Source: CAD feature listing. Evaluate the final solid. Frame: model axes, mm. A direction names the side the tool comes from. Coordinates: 2 decimals unless noted, no trailing zeros. Write each loop counter-clockwise with the first axis right and the second up, starting at its lowest first coordinate (ties: lowest second). Pieces come first, ordered by that corner, then holes. Notation, with made-up numbers: M 52.25,81 L 62.25,81 A16 ccw 62.25,107 Z; hole C 86.25,38 d5. An arc over 180 degrees is marked long. One line per item, written item: value. Start each with the question number.
Item 1: Cut plane B-B, the plane y = 30.25. Output: boundary loops of the cut face in (x, z) (3 decimals), then the cut area to 3 significant figures.
Item 2: Cut plane A-A, the plane x = 0. State how many separate pieces and enclosed holes the cut face has, then the cut area to 3 significant figures.
Item 3: Mould query, pull axis Z, two halves, no side actions, for faces 1 (the cylindrical face through (1, 26, 0)), 2 (the cylindrical face through (2.4, 30.7, -0.5)), 3 (the flat face through (3, 23.4, 0)). Classes: released by +Z, released by -Z, zero draft, split by the parting line, or undercut.
Item 4: Ray query, L1, parallel to Z at x = 0, y = 20.2; L2, parallel to Z at x = 0, y = 29.5; L3, parallel to Z at x = 0, y = 26 (3 decimals). Return the intervals inside material, ascending. Write a range as from..to.
Item 5: Cut plane C-C, the plane y = 22.5. Output: boundary loops of the cut face in (x, z), then the cut area to 3 significant figures.
Item 6: Pin query (flat end, axial travel): P1, Ø2, axis at x = -5, z = 0, coming from the +Y side; P2, Ø1.1, axis at x = 0, z = 5, coming from the +Y side; P3, Ø4, axis at y = 21, z = -4, coming from the +X side; P4, Ø2, axis at y = 22.5, z = -3, coming from the -X side. Return the tip coordinate at first contact, or that it passes through.
Item 7: Set-up query: faces 4 (the cylindrical face through (2.4, 28.2, -0.5)), 5 (the cylindrical face through (-1.792, 30.094, 1.142)), 6 (the cylindrical face through (-2.85, 19.59, -0.37)). Return all of +Z, -Z, +X, -X, +Y, -Y with unobstructed straight access to the full face (end or side cutting, diameter ignored); none if empty.
Item 8: Cut plane D-D, the plane y = 24. Output: boundary loops of the cut face in (x, z), then the cut area to 3 significant figures.
Autodesk Inventor part; units mm, degrees
ref_plane "Work Plane8" through (0, 26.3, 0) normal (0, 1, 0) x (1, 0, 0)
ref_plane "Work Plane9" through (0, 30.1, 0) normal (0, 1, 0) x (1, 0, 0)
ref_plane "YZ Plane" through (0, 0, 0) normal (1, 0, 0) x (0, 1, 0)
sketch "Sketch1" plane through (0, 0, 0) normal (1, 0, 0) x (0, 1, 0)
  line L0 (31, 0) -> (20.4, 0)
  line L1 (31, 0) -> (32, 0)
  line L2 (32, 0) -> (32, 2.45)
  line L3 (32, 2.45) -> (30.5, 2.45)
  line L4 (30.5, 2.45) -> (30.5, 2.125)
  line L5 (30.5, 2.125) -> (29.7, 2.125)
  line L6 (29.7, 2.125) -> (29.7, 2.45)
  line L7 (29.7, 2.45) -> (26.7, 2.45)
  line L8 (26.7, 2.45) -> (26.7, 2.125)
  line L9 (26.7, 2.125) -> (25.9, 2.125)
  line L10 (25.9, 2.125) -> (25.9, 2.45)
  line L11 (25.9, 2.45) -> (24.4, 2.45)
  line L12 (23.4, 2.5) -> (24.4, 2.5)
  line L13 (24.4, 2.5) -> (24.4, 2.45)
  line L14 (23.4, 2.5) -> (23.4, 7.5)
  line L15 (32, 2.45) -> (31, 2.45)
  line L16 (32, 2.45) -> (32, 1.45)
  line L17 (19.6, 7.5) -> (23.4, 7.5)
  line L18 (20.4, 2.55) -> (20, 2.55)
  line L19 (19.2, 7.5) -> (19.6, 7.5)
  line L20 (20.4, 2.55) -> (20.4, 0)
  line L21 (20, 2.55) -> (20, 2.875)
  line L22 (20, 2.875) -> (19.2, 2.875)
  line L23 (19.2, 2.875) -> (19.2, 7.5)
  point P0 (0, 0)
  dimension "d344" = 1
  dimension "d345" = 1.5
  dimension "d346" = 0.325
  dimension "d347" = 0.8
  dimension "d348" = 3
  dimension "d349" = 0.325
  dimension "d350" = 0.8
  dimension "d351" = 2.45
  dimension "d353" = 1
  dimension "d354" = 1
  dimension "d355" = 1
  dimension "d377" = 0.4
  dimension "d379" = 2.55
  dimension "d380" = 0.8
revolve "Revolution1" add sketch "Sketch1" angle 360 about axis through (0, 31, 0) along (0, -1, 0)
chamfer "Chamfer6" distance 0.5 angle 45 2 edges at (0, 23.4, -7.5) (0, 19.2, -7.5)
chamfer "Chamfer8" distance 1 angle 45 1 edges at (0, 32, -2.45)
sketch "Sketch13" plane through (0, 32, 0) normal (0, 1, 0) x (1, 0, 0)
  circle A0 centre (0, 0) radius 1
  point P0 (0, 0)
  dimension "d359" = 2
hole "Hole10" at (0, 32, 0) direction (0, -1, 0) diameter 2 end through all
ref_plane "Work Plane8" through (0, 26.3, 0) normal (0, 1, 0) x (1, 0, 0)
ref_plane "Work Plane9" through (0, 30.1, 0) normal (0, 1, 0) x (1, 0, 0)
sketch "Sketch15" plane through (0, 19.2, 0) normal (0, -1, 0) x (1, 0, 0)
  line L0 (0, 0) -> (5, 0)
  line L1 (0, 0) -> (-5, 0)
  line L2 (0, 0) -> (0, -5)
  line L3 (0, 0) -> (0, 5)
  dimension "d381" = 5
  dimension "d382" = 5
  dimension "d383" = 5
  dimension "d384" = 5
hole "Hole11" at (0, 19.2, -5) at (-5, 19.2, 0) at (5, 19.2, 0) at (0, 19.2, 5) direction (0, 1, 0) diameter 1.9 end through all
thread "Thread21"
thread "Thread22"
thread "Thread23"
thread "Thread24"
properties part number "None_Magnet_Extender_Split_Top" material "Aluminum 6061"
From the geometry:
1. outline: C 0,0 d4.25; hole C 0,0 d2
1. area: 11.0 mm²
2. separate pieces: 4
2. enclosed holes: 0
2. area: 56.9 mm²
3. face 1: undercut
3. face 2: split by the parting line
3. face 3: zero draft
4. L1: z = -7.5..-5.95, -4.05..-2.55, 2.55..4.05, 5.95..7.5
4. L2: z = -2.45..-1, 1..2.45
4. L3: z = -2.125..-1, 1..2.125
5. outline: C 0,0 d15; hole C -5,0 d1.9; hole C 0,0 d2; hole C 0,-5 d1.9; hole C 0,5 d1.9; hole C 5,0 d1.9
5. area: 162 mm²
6. P1: stops at y = 23.4
6. P2: passes through
6. P3: stops at x = 7.23
6. P4: stops at x = -7.23
7. face 4: +Y
7. face 5: none
7. face 6: -Y
8. outline: C 0,0 d5; hole C 0,0 d2
8. area: 16.5 mm²
